Design review of the part built by this model. Coordinates are the model's own, in mm. A direction names the side the tool comes from. Coordinates: 2 decimals unless noted, no trailing zeros. Order: outer loops, then holes, each group sorted by start corner. A loop starts at its lowest first (then second) coordinate and runs counter-clockwise, first axis right, second up. Notation, with made-up numbers: M 78.25,65.5 L 116.25,65.5 A16 cw 116.25,73.5 Z; hole C 68,-35 d6. An arc over 180 degrees is marked long. Answer as a JSON object with one key per item and string values.
Autodesk Inventor part; units mm, degrees
ref_plane "YZ Plane" through (0, 0, 0) normal (1, 0, 0) x (0, 1, 0)
ref_plane "XZ Plane" through (0, 0, 0) normal (0, 1, 0) x (-1, 0, 0)
ref_plane "XY Plane" through (0, 0, 0) normal (0, 0, 1) x (1, 0, 0)
sketch "Sketch1" plane through (0, 0, 0) normal (0, 0, 1) x (1, 0, 0)
  line L0 (-19.05, -19.05) -> (19.05, -19.05)
  line L1 (19.05, -19.05) -> (19.05, 19.05)
  line L2 (19.05, 19.05) -> (-19.05, 19.05)
  line L3 (-19.05, 19.05) -> (-19.05, -19.05)
  line L4 (-19.05, -19.05) -> (19.05, 19.05) construction
  line L5 (19.05, -19.05) -> (-19.05, 19.05) construction
  line L6 (14.2875, -14.2875) -> (-14.2875, -14.2875) construction
  line L7 (-14.2875, -14.2875) -> (-14.2875, 14.2875) construction
  line L8 (-14.2875, 14.2875) -> (14.2875, 14.2875) construction
  line L9 (14.2875, 14.2875) -> (14.2875, -14.2875) construction
  line L10 (14.2875, -14.2875) -> (-14.2875, 14.2875) construction
  line L11 (-14.2875, -14.2875) -> (14.2875, 14.2875) construction
  circle A0 centre (0, 0) radius 12.7
  circle A1 centre (0, 0) radius 12
  circle A2 centre (0, 0) radius 9.525
  dimension "d0" = 38.1
  dimension "d1" = 38.1
  dimension "d3" = 25.4
  dimension "d4" = 24
  dimension "d5" = 19.05
  dimension "d20" = 28.575
extrude "Extrusion1" add sketch "Sketch1" against normal blind 9.525 contours L3 L2 L1 L0 | A0 | A1
extrude "Extrusion2" cut sketch "Sketch1" against normal blind 2.1906 contours A0
extrude "Extrusion3" cut sketch "Sketch1" against normal blind 8.1906 contours A1
hole "Hole1" at (-14.2875, 14.2875, 0) at (14.2875, 14.2875, 0) at (14.2875, -14.2875, 0) at (-14.2875, -14.2875, 0) direction (0, 0, -1) diameter 4.318 end through all
sketch "Sketch2" plane through (0, 0, -9.525) normal (0, 0, -1) x (-1, 0, 0)
  line L0 (-19.05, -19.05) -> (19.05, -19.05)
  line L1 (19.05, -19.05) -> (19.05, 19.05)
  line L2 (19.05, 19.05) -> (-19.05, 19.05)
  line L3 (-19.05, 19.05) -> (-19.05, -19.05)
  circle A0 centre (-14.2875, -14.2875) radius 2.159
  circle A1 centre (14.2875, 14.2875) radius 2.159
  circle A2 centre (-14.2875, 14.2875) radius 2.159
  circle A3 centre (14.2875, -14.2875) radius 2.159
  circle A4 centre (0, 0) radius 9.525
  circle A5 centre (-14.2875, 14.2875) radius 3.429 construction
  circle A6 centre (0, 0) radius 12 construction
  circle A7 centre (0, 0) radius 15.0812
  dimension "d21" = 6.858
  dimension "d22" = 24
  dimension "d23" = 30.1625
extrude "Extrusion4" cut sketch "Sketch2" against normal blind 3.175 contours L3 L2 L1 L0
equation "\"d1\" = d0"
properties part number "Module Top Cap"
1) Insertion check: pin 1 Ø1.5 at (y, z) = (-7, -7.5) entering from +X; pin 2 Ø5 at (x, y) = (-14.29, -14.29) entering from -Z; pin 3 Ø1 at (x, z) = (12.5, -7) entering from -Y. Each pin has a flat end and moves straight along its axis. Give the tip position at first contact, or say it passes through.
Taken from the geometry:
{"pin 1": "stops at x = 13.73", "pin 2": "stops at z = -6.35", "pin 3": "stops at y = -9.13"}
2) Add section B-B (x = 1). State the section outline as (y, z) points (3 decimals), and give its area (3 significant figures).
Taken from the geometry:
{"outline": "M -19.05,-6.35 L -15.048,-6.35 L -15.048,-9.525 L -9.472,-9.525 L -9.472,-8.191 L -11.958,-8.191 L -11.958,-2.191 L -12.661,-2.191 L -12.661,0 L -19.05,0 Z; M 9.472,-9.525 L 15.048,-9.525 L 15.048,-6.35 L 19.05,-6.35 L 19.05,0 L 12.661,0 L 12.661,-2.191 L 11.958,-2.191 L 11.958,-8.191 L 9.472,-8.191 Z", "area": "113 mm2"}
3) Mouldability with a two-part tool opening along X and no side actions: class faces 1 (the flat face through (0, 13, 0)), 2 (the flat face through (-19.05, 0, -3)), 3 (the cylindrical face through (13.639, -16.347, -3.219)) as released by +X, released by -X, zero draft, split by the parting line, or undercut.
Taken from the geometry:
{"face 1": "zero draft", "face 2": "released by -X", "face 3": "undercut"}
4) Add section D-D (z = -7.75). State the section outline as (x, y) points, and give its area (3 significant figures).
Taken from the geometry:
{"outline": "C 0,0 d30.16; hole C 0,0 d24", "area": "262 mm2"}
5) Add section A-A (y = 0). State the section outline as (x, z) points (3 decimals).
Taken from the geometry:
{"outline": "M -19.05,-6.35 L -15.081,-6.35 L -15.081,-9.525 L -9.525,-9.525 L -9.525,-8.191 L -12,-8.191 L -12,-2.191 L -12.7,-2.191 L -12.7,0 L -19.05,0 Z; M 9.525,-9.525 L 15.081,-9.525 L 15.081,-6.35 L 19.05,-6.35 L 19.05,0 L 12.7,0 L 12.7,-2.191 L 12,-2.191 L 12,-8.191 L 9.525,-8.191 Z"}
6) To check wall thickness, follow L1, parallel to Y at x = 0, z = -3.9; L2, parallel to Y at x = 0, z = -8.85 (3 decimals); L3, parallel to X at y = 15.5, z = -0.5. State the ranges of each line that lie inside material, in increasing order.
Taken from the geometry:
{"L1": "y = -19.05 to -12, 12 to 19.05", "L2": "y = -15.081 to -9.525, 9.525 to 15.081", "L3": "x = -19.05 to -16.07, -12.5 to 12.5, 16.07 to 19.05"}
7) Add section C-C (z = -3). State the section outline as (x, y) points, and give its area (3 significant figures).
Taken from the geometry:
{"outline": "M -19.05,-19.05 L 19.05,-19.05 L 19.05,19.05 L -19.05,19.05 Z; hole C -14.29,-14.29 d4.32; hole C -14.29,14.29 d4.32; hole C 0,0 d24; hole C 14.29,-14.29 d4.32; hole C 14.29,14.29 d4.32", "area": "941 mm2"}
8) Tool access review of faces 4 (the flat face through (13, 9, -6.35)), 5 (the flat face through (0, -19.05, -3)), 6 (the cylindrical face through (-11.99, 0.53, -5.15)): name each direction out of +Z, -Z, +X, -X, +Y, -Y from which nothing blocks a thin tool from reaching the whole face with its end or side.
Taken from the geometry:
{"face 4": "-Z", "face 5": "+Z, -Z, +X, -X, -Y", "face 6": "+Z"}
